Geometry check sheet. Reference: the model listing, model coordinates, mm. A direction names the side the tool comes from. Coordinates: 2 decimals unless noted, no trailing zeros. Write each loop counter-clockwise with the first axis right and the second up, starting at its lowest first coordinate (ties: lowest second). Pieces come first, ordered by that corner, then holes. Notation, with made-up numbers: (-8, 66) -> (42, 66) arc R23 ccw to (42, 76) -> close; hole circle Ø8 at (-6, 70). An arc over 180 degrees is marked (long way). Use a Markdown table: item, result.
Autodesk Inventor part; units mm, degrees
ref_plane "YZ Plane" through (0, 0, 0) normal (1, 0, 0) x (0, 1, 0)
ref_plane "XZ Plane" through (0, 0, 0) normal (0, 1, 0) x (-1, 0, 0)
ref_plane "XY Plane" through (0, 0, 0) normal (0, 0, 1) x (1, 0, 0)
sketch "Sketch1" plane through (0, 0, 0) normal (0, 0, 1) x (1, 0, 0)
  line L0 (0, 0) -> (-74, 0)
  line L1 (-74, 0) -> (-74, 10)
  line L2 (-74, 10) -> (0, 10)
  line L3 (0, 10) -> (0, 0)
  line L4 (-74, 10) -> (-64, 0) construction
  line L5 (0, 10) -> (-10, 0) construction
  circle A0 centre (-69, 5) radius 4
  circle A1 centre (-5, 5) radius 4
  circle A2 centre (-69, 5) radius 1.45
  circle A3 centre (-5, 5) radius 1.45
  line L6 (0, -64) -> (-74, -64)
  line L7 (-74, -64) -> (-74, -54)
  line L8 (-74, -54) -> (0, -54)
  line L9 (0, -54) -> (0, -64)
  line L10 (-74, -54) -> (-64, -64) construction
  line L11 (0, -54) -> (-10, -64) construction
  circle A4 centre (-69, -59) radius 4
  circle A5 centre (-5, -59) radius 4
  circle A6 centre (-69, -59) radius 1.45
  circle A7 centre (-5, -59) radius 1.45
  line L12 (-74, -54) -> (-69, -54)
  line L13 (-69, -54) -> (-69, 0)
  line L14 (-69, 0) -> (-74, 0)
  line L15 (-74, 0) -> (-74, -54)
  line L16 (0, -54) -> (-5, -54)
  line L17 (-5, -54) -> (-5, 0)
  line L18 (-5, 0) -> (0, 0)
  line L19 (0, 0) -> (0, -54)
  point P0 (-5, 0)
  point P1 (-69, -54)
  dimension "d0" = 74
  dimension "d1" = 10
  dimension "d2" = 45
  dimension "d3" = 8
  dimension "d5" = 2.9
  dimension "d22" = 74
  dimension "d23" = 5
extrude "Extrusion1" add sketch "Sketch1" against normal blind 3 contours L0 L1 L2 L3 | L9 L6 L7 L8 | A0 | A1 | A2 | A3 | A4 | A5 | A6 | A7
extrude "Extrusion2" add sketch "Sketch1" against normal blind 29 contours A0 | A1 | A4 | A5
extrude "Extrusion3" add sketch "Sketch1" against normal blind 0.5 contours L19 L8 L17 L0 | L13 L8 L15 L0
fillet "Fillet1" radius 2 8 edges at (-74, 10, -1.5) (-74, 0, -1.75) (0, 10, -1.5) (0, 0, -1.75) (-74, -54, -1.75) (-74, -64, -1.5) (0, -54, -1.75) (0, -64, -1.5)
chamfer "Chamfer1" distance 0.25 angle 45 34 edges at (-37, 10, -3) (-0.5858, 9.4142, -3) (0, 5, -3) (-0.5858, 0.5858, -3) (-37, 0, -3) (-73.4142, 0.5858, -3) (-74, 5, -3) (-73.4142, 9.4142, -3) (-37, 0, 0) (-9, 5, -29) (-6.45, 5, -29) (-73, 5, -29) (-70.45, 5, -29) (-37, -54, -3) (-0.5858, -54.5858, -3) (0, -59, -3) (-0.5858, -63.4142, -3) (-37, -64, -3) (-73.4142, -63.4142, -3) (-74, -59, -3) (-73.4142, -54.5858, -3) (-37, -54, 0) (-73, -59, -29) (-70.45, -59, -29) (-9, -59, -29) (-6.45, -59, -29) (-70.5, 0, -0.5) (-3.5, 0, -0.5) (-3.5, -54, -0.5) (-70.5, -54, -0.5) (-6.45, -59, -3) (-6.45, 5, -3) (-70.45, 5, -3) (-70.45, -59, -3)
properties part number "ScanCoverMount"
Item 1: Tool access check on faces 1 (the conical face through (-73.342, -63.312, -2.873)), 2 (the conical face through (-0.658, -54.688, -2.873)), 3 (the cylindrical face through (-70.15, 4.12, -15.82)). Record the directions out of +Z, -Z, +X, -X, +Y, -Y that give a thin tool (end or side, any length) a straight path to the whole face; none if there is none.
Answer block:
| item | result |
|---|---|
| face 1 | -Z, -X, -Y |
| face 2 | -Z, +X |
| face 3 | -Z |
Item 2: Mould release check, pull along Y, two halves, no side actions. Record for faces 4 (the conical face through (-73.312, 9.342, -2.873)), 5 (the flat face through (-4, 3, -29)), 6 (the flat face through (-72, -27, -0.5)), 7 (the flat face through (-69, -59, -3)): +Y half, -Y half, draft (parallel to the pull), parting line (faces both ways), or undercut.
Answer block:
| item | result |
|---|---|
| face 4 | +Y half |
| face 5 | draft |
| face 6 | undercut |
| face 7 | undercut |
Item 3: Section check B-B on x = -35.5. Record the boundary of the cut face in (y, z).
Answer block:
| item | result |
|---|---|
| outline | (-64, -2.75) -> (-63.75, -3) -> (-54.25, -3) -> (-54, -2.75) -> (-54, -0.25) -> (-54.25, 0) -> (-64, 0) -> close; (0, -2.75) -> (0.25, -3) -> (9.75, -3) -> (10, -2.75) -> (10, 0) -> (0.25, 0) -> (0, -0.25) -> close |
Item 4: Section check D-D on y = -29.5. Record the boundary of the cut face in (x, z), then the cut area to 3 significant figures.
Answer block:
| item | result |
|---|---|
| outline | (-74, -0.5) -> (-69, -0.5) -> (-69, 0) -> (-74, 0) -> close; (-5, -0.5) -> (0, -0.5) -> (0, 0) -> (-5, 0) -> close |
| area | 5.00 mm^2 |
Item 5: Section check A-A on z = -20.5. Record the boundary of the cut face in (x, y).
Answer block:
| item | result |
|---|---|
| outline | circle Ø8 at (-69, -59); circle Ø8 at (-69, 5); circle Ø8 at (-5, -59); circle Ø8 at (-5, 5); hole circle Ø2.9 at (-69, -59); hole circle Ø2.9 at (-69, 5); hole circle Ø2.9 at (-5, -59); hole circle Ø2.9 at (-5, 5) |
Item 6: Depth check by flat-ended pin: P1, Ø2.5, axis at x = -5.5, y = -59.5, coming from the -Z side; P2, Ø10, axis at x = -16, y = -53, coming from the -Z side; P3, Ø5.5, axis at x = -71.5, y = -21.5, coming from the -Z side; P4, Ø2.5, axis at x = -5, y = 5, coming from the -Z side. Enter the tip coordinate at first touch or a pass-through.
Answer block:
| item | result |
|---|---|
| P1 | stops at z = -29 |
| P2 | stops at z = -3 |
| P3 | stops at z = -0.5 |
| P4 | stops at z = -3.05 |
Item 7: Thickness scan on L1, parallel to Y at x = -5, z = -10.5; L2, parallel to Y at x = -54, z = -1.25; L3, parallel to Z at x = -49.5, y = -57.5. Record the ranges inside material, lowest first. Write a range as [from, to].
Answer block:
| item | result |
|---|---|
| L1 | y = [-63, -60.45], [-57.55, -55], [1, 3.55], [6.45, 9] |
| L2 | y = [-64, -54], [0, 10] |
| L3 | z = [-3, 0] |
